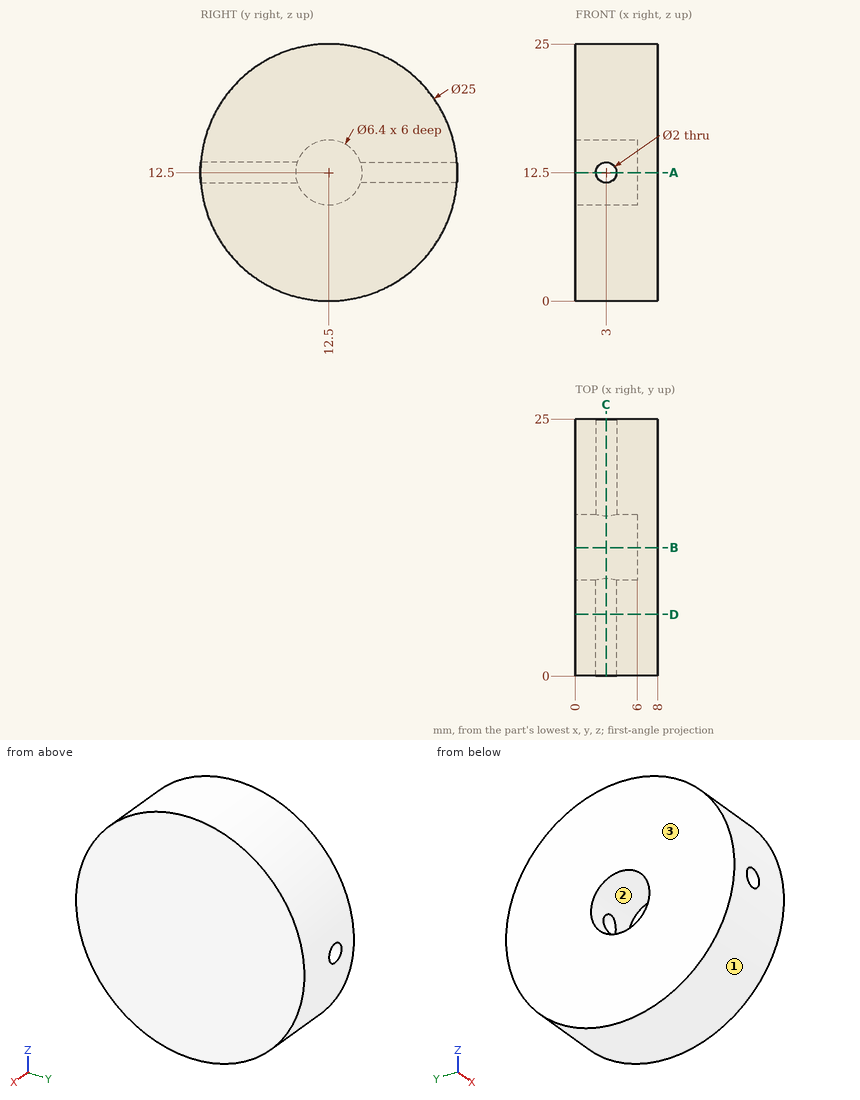
The drawing under review shows one solid part. Ordinate dimensions are in mm from its lowest x, y, z. Coordinates: 2 decimals unless noted, no trailing zeros. Write each loop counter-clockwise with the first axis right and the second up, starting at its lowest first coordinate (ties: lowest second). Pieces come first, ordered by that corner, then holes.
1) Add section B-B (y = 12.5). Write out the cut boundary in (x, z), plus the area to 3 significant figures.
2) Insertion check: pin 1 (3 mm diameter, centred on y = 14, z = 11.5, fed in from -X); pin 2 (1.5 mm diameter, centred on x = 2.5, z = 19, fed in from +Y); pin 3 (3 mm diameter, centred on x = 5.5, y = 9, fed in from +Z). Each pin has a flat end and moves straight along its axis. Give the tip position at first contact, or say it passes through.
3) Add section A-A (z = 12.5). Write out the cut boundary in (x, y).
4) Add section C-C (x = 3). Write out the cut boundary in (y, z), plus the area to 3 significant figures.
5) To check wall thickness, follow L1, parallel to Y at x = 1.5, z = 12.5; L2, parallel to X at y = 5.5, z = 12.5; L3, parallel to Z at x = 3, y = 11.5. State the ranges of each line that lie inside material, in increasing order.
6) Add section D-D (y = 6). Write out the cut boundary in (x, z).
7) Mouldability with a two-part tool opening along Y and no side actions: class the marked faces 1, 2 and 3 as +Y half, -Y half, draft (parallel to the pull), parting line (faces both ways), or undercut.
Check result:
1. outline: (0, 0) - (8, 0) - (8, 25) - (0, 25) - (0, 15.7) - (6, 15.7) - (6, 9.3) - (0, 9.3) - close
1. area: 162 mm2
2. pin 1: stops at x = 0
2. pin 2: stops at y = 23.6
2. pin 3: stops at z = 24.84
3. outline: (0, 0) - (2, 0) - (2, 9.3) - (0, 9.3) - close; (0, 15.7) - (2, 15.7) - (2, 25) - (0, 25) - close; (4, 0) - (8, 0) - (8, 25) - (4, 25) - (4, 15.7) - (6, 15.7) - (6, 9.3) - (4, 9.3) - close
4. outline: (0.04, 11.5) arc R12.5 ccw to (24.96, 11.5) - (15.54, 11.5) arc R3.2 cw to (9.46, 11.5) - close; (0.04, 13.5) - (9.46, 13.5) arc R3.2 cw to (15.54, 13.5) - (24.96, 13.5) arc R12.5 ccw to start
4. area: 421 mm2
5. L1: y = 0 to 9.3, 15.7 to 25
5. L2: x = 0 to 2, 4 to 8
5. L3: z = 0.04 to 9.46, 15.54 to 24.96
6. outline: (0, 1.82) - (8, 1.82) - (8, 23.18) - (0, 23.18) - close; hole circle Ø2 at (3, 12.5)
7. face 1: parting line
7. face 2: undercut
7. face 3: draft
